Check sheet for the modelled part. Datum: model origin and axes. Units: mm. Give positions to 0.01 mm unless a question says otherwise; leave off trailing zeros. Write each loop counter-clockwise with the first axis right and the second up, starting at its lowest first coordinate (ties: lowest second). Pieces come first, ordered by that corner, then holes. Notation, with made-up numbers: M 73,85 L 79,85 A17 cw 79,97 Z; hole C -2,-20.75 d6. An arc over 180 degrees is marked long. Write item = value, one per line. Start each with the question number.
1) Cross-section at D-D, the plane z = -6.35. Record the cut outline in (x, y) (1 decimal).
2) Cross-section at C-C, the plane x = -12.7. Record the cut outline in (y, z) (3 decimals).
3) Scan lines: line 1 along X through (y, z) = (1.3, 12.7); line 2 along Z through (x, y) = (0, 2.4); line 3 along Z through (x, y) = (-46.5, 0.35). Record each from-to range of solid material in increasing order. Write a range as [from, to].
4) Cross-section at A-A, the plane z = 12.7. Record the cut outline in (x, y) (1 decimal).
5) Go/stop test with a flat-tipped pin: pin 1 (4 mm diameter, centred on x = 46.04, z = 12.7, fed in from +Y). Record where the tip stops, or that it passes through.
6) Cross-section at B-B, the plane x = 57.15. Record the cut outline in (y, z) (3 decimals).
7) Mould release check, pull along Z, two halves, no side actions. Record for faces 1 (the cylindrical face through (-47.27, 1.57, 53.98)), 2 (the flat face through (-1, 2, -57.15)), 3 (the flat face through (-61.912, 2, 1)), 4 (the flat face through (-1, 2, 57.15)): released by +Z, released by -Z, zero draft, split by the parting line, or undercut.
```python
from build123d import *

# Parameters (mm, degrees)
SKETCH1_W                                = 123.825
SKETCH1_H                                = 114.3
PLATE_DEPTH                              = 3.175
FORCE_PLATE_POST_1_4_20_CLEARANCE_HOLE_D = 6.7564
F_4_CLEARANCE_HOLE1_D                    = 3.2639
F_10_CLEARANCE_HOLE1_D                   = 5.1054


with BuildPart() as part:
    # Sketch1 → Plate (new body)
    with BuildSketch(Plane(origin=(0, 0, 0), x_dir=(1, 0, 0), z_dir=(0, 1, 0))):
        Rectangle(SKETCH1_W, SKETCH1_H)
    extrude(amount=PLATE_DEPTH)

    # Force Plate Post (1/4"-20 Clearance Hole) (through all)
    with Locations(Plane(origin=(0, 3.175, 0), x_dir=(1, 0, 0), z_dir=(0, 1, 0))):
        with Locations((0, 6.35)):
            Hole(FORCE_PLATE_POST_1_4_20_CLEARANCE_HOLE_D / 2)

    # #4 Clearance Hole1 (through all)
    with Locations(Plane(origin=(0, 3.175, 0), x_dir=(1, 0, 0), z_dir=(0, 1, 0))):
        with Locations((57.15, -52.3875), (57.15, -17.4625), (57.15, 17.4625), (22.225, -52.3875), (-12.7, -52.3875), (-47.625, -52.3875)):
            Hole(F_4_CLEARANCE_HOLE1_D / 2)

    # #10 Clearance Hole1 (through all)
    with Locations(Plane(origin=(0, 3.175, 0), x_dir=(1, 0, 0), z_dir=(0, 1, 0))):
        with Locations((0, 41.275), (-46.0375, -12.7), (46.0375, -12.7)):
            Hole(F_10_CLEARANCE_HOLE1_D / 2)


solid = part.part
```
Reply:
q1.outline = M -61.9,0 L -3.4,0 L -3.4,3.2 L -61.9,3.2 Z; M 3.4,0 L 61.9,0 L 61.9,3.2 L 3.4,3.2 Z
q2.outline = M 0,-57.15 L 3.175,-57.15 L 3.175,50.756 L 0,50.756 Z; M 0,54.019 L 3.175,54.019 L 3.175,57.15 L 0,57.15 Z
q3.line_1 = [-61.91, -48.59], [-43.48, 43.48], [48.59, 61.91]
q3.line_2 = [-57.15, -43.83], [-38.72, -9.73], [-2.97, 57.15]
q3.line_3 = [-57.15, 10.19], [15.21, 51.21], [53.57, 57.15]
q4.outline = M -61.9,0 L -48.6,0 L -48.6,3.2 L -61.9,3.2 Z; M -43.5,0 L 43.5,0 L 43.5,3.2 L -43.5,3.2 Z; M 48.6,0 L 61.9,0 L 61.9,3.2 L 48.6,3.2 Z
q5.pin_1 = through
q6.outline = M 0,-57.15 L 3.175,-57.15 L 3.175,-19.094 L 0,-19.094 Z; M 0,-15.831 L 3.175,-15.831 L 3.175,15.831 L 0,15.831 Z; M 0,19.094 L 3.175,19.094 L 3.175,50.756 L 0,50.756 Z; M 0,54.019 L 3.175,54.019 L 3.175,57.15 L 0,57.15 Z
q7.face_1 = undercut
q7.face_2 = released by -Z
q7.face_3 = zero draft
q7.face_4 = released by +Z
